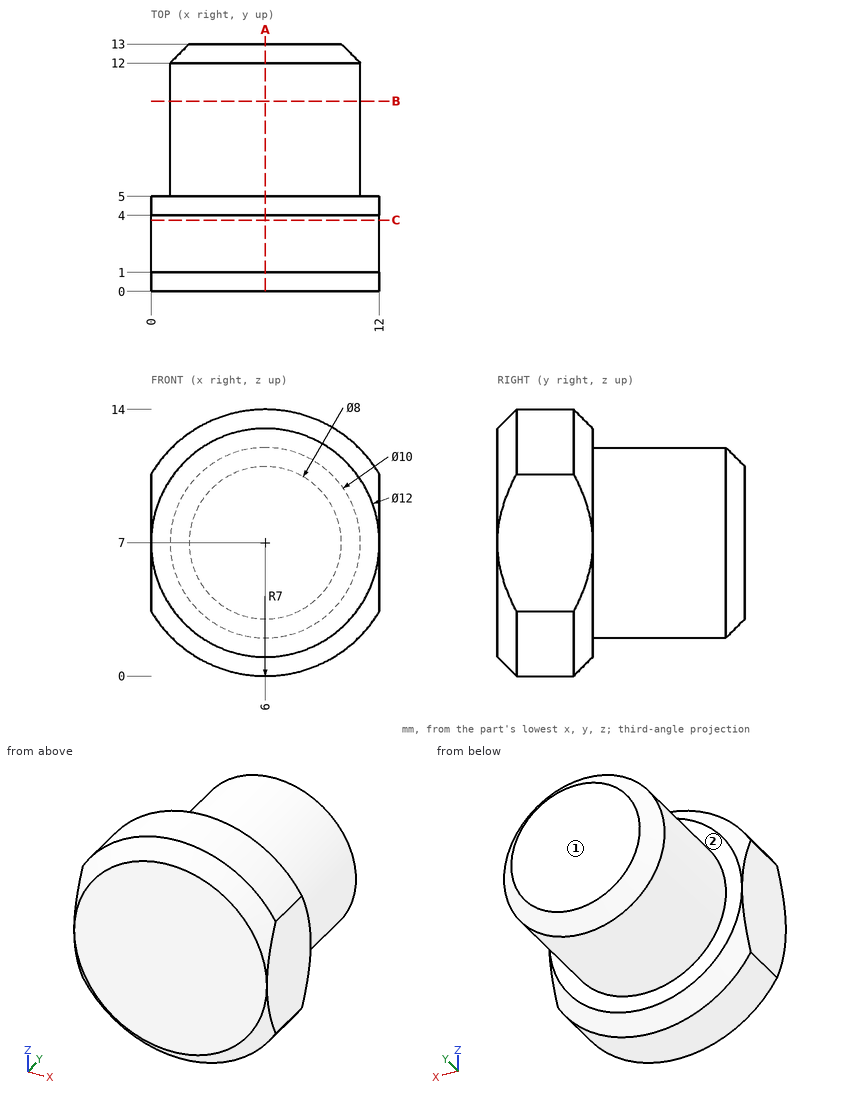
Geometry: see drawing. Coordinates: mm, zero at the bounding-box minimum. A direction names the side the tool comes from. Coordinates: 2 decimals unless noted, no trailing zeros. Loops run counter-clockwise (first coordinate to the right, second up) from the corner with the lowest first, then second, coordinate; pieces in that order, holes last. Notation, with made-up numbers: M -38.5,-38 L -9.5,-38 A19 cw -9.5,-7 Z; hole C 89.25,50 d3. An arc over 180 degrees is marked long. Answer in a Markdown table with one row per item.
1. Material intervals for line 1 (Y direction, x = 4.25, z = 1.5); line 2 (X direction, y = 11, z = 4); line 3 (Z direction, x = 10, y = 6.5), sorted ascending.
Response:
| item | result |
|---|---|
| line 1 | y = 0 to 5 |
| line 2 | x = 2 to 10 |
| line 3 | z = 4 to 10 |
2. First-contact query: pin 1 (2 mm diameter, centred on x = 4.5, y = 5, fed in from -Z); pin 2 (1.5 mm diameter, centred on y = 9.5, z = 5.5, fed in from -X); pin 3 (5 mm diameter, centred on x = 5, y = 9.5, fed in from -Z). Flat tips, straight axial feed; report the tip coordinate or a pass-through.
Response:
| item | result |
|---|---|
| pin 1 | stops at z = 0.14 |
| pin 2 | stops at x = 1.06 |
| pin 3 | stops at z = 2 |
3. Section C-C, the plane y = 3.75. Output: boundary loops of the cut face in (x, z).
Response:
| item | result |
|---|---|
| outline | M 0,3.39 A7 ccw 12,3.39 L 12,10.61 A7 ccw 0,10.61 Z |
4. Reachability of the marked faces 1 and 2 from +Z, -Z, +X, -X, +Y, -Y: full face, straight path, thin tool, end or side. Return the list, or none.
Response:
| item | result |
|---|---|
| face 1 | +Z, -Z, +X, -X, +Y |
| face 2 | +Y |
5. Section B-B, the plane y = 10. Output: boundary loops of the cut face in (x, z), then the cut area to 3 significant figures.
Response:
| item | result |
|---|---|
| outline | C 6,7 d10 |
| area | 78.5 mm2 |
6. Section A-A, the plane x = 6. Output: boundary loops of the cut face in (y, z).
Response:
| item | result |
|---|---|
| outline | M 0,1 L 1,0 L 4,0 L 5,1 L 5,2 L 12,2 L 13,3 L 13,11 L 12,12 L 5,12 L 5,13 L 4,14 L 1,14 L 0,13 Z |
